Work out the finished part from the listing and answer in its coordinate system (mm). Coordinates: 2 decimals unless noted, no trailing zeros. Loops run counter-clockwise (first coordinate to the right, second up) from the corner with the lowest first, then second, coordinate; pieces in that order, holes last. Notation, with made-up numbers: (83.25, 28) -> (103.25, 28) arc R25 ccw to (103.25, 47) -> close; hole circle Ø3 at (-10, -19). An arc over 180 degrees is marked (long way). Use a Markdown table: item, result.
from build123d import *

# Parameters (mm, degrees)
SKETCH_1_W          = 56
SKETCH_1_H          = 35
EXTRUDE_1_DEPTH     = 5
SKETCH_3_R          = 1.5
CUT_EXTRUDE_1_DEPTH = 10
FILLET_1_R          = 6


with BuildPart() as part:
    # Эскиз1 → Бобышка-Вытянуть1 (new body)
    with BuildSketch(Plane(origin=(0, 0, 0), x_dir=(1, 0, 0), z_dir=(0, 1, 0))):
        Polygon((-31.5, -31), (-82.5, -31), (-82.5, 21), (-82.5, 31), (31.5, 31), (31.5, -31), align=None)
        with Locations((-10.5, -0.5)):
            Rectangle(SKETCH_1_W, SKETCH_1_H, mode=Mode.SUBTRACT)
    extrude(amount=EXTRUDE_1_DEPTH)

    # Эскиз3 → Вырез-Вытянуть1 (cut)
    with BuildSketch(Plane.XZ):
        with Locations(Location((15.5, 21, 0), (0, 0, 270))):
            Circle(SKETCH_3_R)
        with Locations(Location((15.5, -21, 0), (0, 0, 270))):
            Circle(SKETCH_3_R)
        with Locations(Location((-77.5, 21, 0), (0, 0, 270))):
            Circle(SKETCH_3_R)
        with Locations(Location((-77.5, -21, 0), (0, 0, 270))):
            Circle(SKETCH_3_R)
    extrude(amount=-CUT_EXTRUDE_1_DEPTH, mode=Mode.SUBTRACT)

    # Скругление1
    fillet_1_edges = [part.edges().sort_by_distance(p)[0] for p in [
        (-82.5, 2.5, 31),
        (-82.5, 2.5, -31),
        (31.5, 2.5, -31),
        (31.5, 2.5, 31),
    ]]
    fillet(fillet_1_edges, radius=FILLET_1_R)


solid = part.part
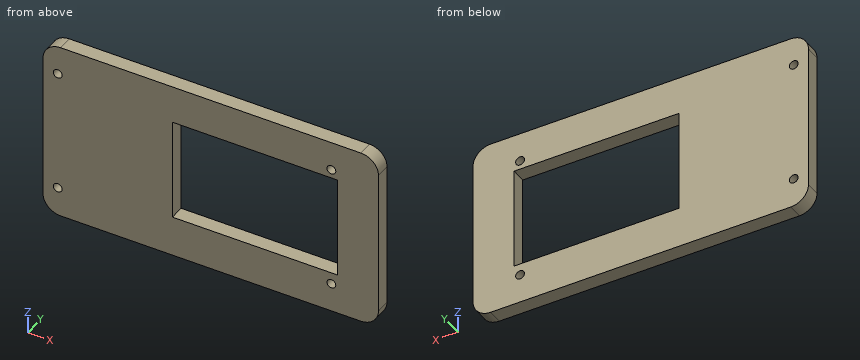
Q1. Consider line 1 (X direction, y = 3.6, z = 21); line 2 (Z direction, x = -10.5, y = 2.25); line 3 (X direction, y = 4.1, z = 1). Determine where each line is inside the solid, lowest interval first. Write a range as [from, to].
Solved:
| item | result |
|---|---|
| line 1 | [-82.5, -79], [-76, 14], [17, 31.5] |
| line 2 | [-31, -17], [18, 31] |
| line 3 | [-82.5, -38.5], [17.5, 31.5] |
Q2. Section B-B on y = 3.15 is taken. Determine the outline of the cut face in (x, z).
Solved:
| item | result |
|---|---|
| outline | (-82.5, -25) arc R6 ccw to (-76.5, -31) -> (25.5, -31) arc R6 ccw to (31.5, -25) -> (31.5, 25) arc R6 ccw to (25.5, 31) -> (-76.5, 31) arc R6 ccw to (-82.5, 25) -> close; hole circle Ø3 at (-77.5, -21); hole circle Ø3 at (-77.5, 21); hole (-38.5, -17) -> (17.5, -17) -> (17.5, 18) -> (-38.5, 18) -> close; hole circle Ø3 at (15.5, -21); hole circle Ø3 at (15.5, 21) |
Q3. Section C-C on z = -13.5 is taken. Determine the outline of the cut face in (x, y), and give its area (3 significant figures).
Solved:
| item | result |
|---|---|
| outline | (-82.5, 0) -> (-38.5, 0) -> (-38.5, 5) -> (-82.5, 5) -> close; (17.5, 0) -> (31.5, 0) -> (31.5, 5) -> (17.5, 5) -> close |
| area | 290 mm² |
Q4. Section D-D on x = -20 is taken. Determine the outline of the cut face in (y, z), and give its area (3 significant figures).
Solved:
| item | result |
|---|---|
| outline | (0, -31) -> (5, -31) -> (5, -17) -> (0, -17) -> close; (0, 18) -> (5, 18) -> (5, 31) -> (0, 31) -> close |
| area | 135 mm² |
Q5. Section A-A on x = 15.5 is taken. Determine the outline of the cut face in (y, z).
Solved:
| item | result |
|---|---|
| outline | (0, -31) -> (5, -31) -> (5, -22.5) -> (0, -22.5) -> close; (0, -19.5) -> (5, -19.5) -> (5, -17) -> (0, -17) -> close; (0, 18) -> (5, 18) -> (5, 19.5) -> (0, 19.5) -> close; (0, 22.5) -> (5, 22.5) -> (5, 31) -> (0, 31) -> close |
